from build123d import *

# Parameters (mm, degrees)
CROQUIS1_R              = 2.75
CROQUIS1_R_2            = 1.75
CROQUIS1_R_3            = 1.747778747
CROQUIS1_R_4            = 7.725412866
SALIENTE_EXTRUIR1_DEPTH = 5
CROQUIS2_R              = 3.175
CROQUIS2_R_2            = 27.5
CORTAR_EXTRUIR1_DEPTH   = 5


with BuildPart() as part:
    # Croquis1 → Saliente-Extruir1 (new body)
    with BuildSketch(Plane.XY):
        Polygon((-28.2, -55.083487529), (-28.2, -31.8), (-4.898409704, -31.8), (-4.898409704, 78.2), (5.101590296, 78.2), (5.101590296, -31.8), (28.2, -31.8), (28.2, -54.916512471), (148.2, -54.916512471), (148.2, -64.916512471), (28.2, -64.916512471), (28.2, -88.2), (-28.2, -88.2), (-28.2, -65.083487529), (-148.2, -65.083487529), (-148.2, -55.083487529), align=None)
        with Locations((-23.57, -36.43)):
            Circle(CROQUIS1_R, mode=Mode.SUBTRACT)
        with Locations((23.57, -36.43)):
            Circle(CROQUIS1_R, mode=Mode.SUBTRACT)
        with Locations((23.57, -83.57)):
            Circle(CROQUIS1_R, mode=Mode.SUBTRACT)
        with Locations((-23.57, -83.57)):
            Circle(CROQUIS1_R, mode=Mode.SUBTRACT)
        with Locations((-15.7, -35.3)):
            Circle(CROQUIS1_R_2, mode=Mode.SUBTRACT)
        with Locations((24.7, -44.3)):
            Circle(CROQUIS1_R_3, mode=Mode.SUBTRACT)
        with Locations((15.7, -84.7)):
            Circle(CROQUIS1_R_2, mode=Mode.SUBTRACT)
        with Locations((-24.7, -75.7)):
            Circle(CROQUIS1_R_2, mode=Mode.SUBTRACT)
        with Locations((0, -60)):
            Circle(CROQUIS1_R_4, mode=Mode.SUBTRACT)
    extrude(amount=SALIENTE_EXTRUIR1_DEPTH)

    # Croquis2 → Cortar-Extruir1 (cut)
    with BuildSketch(Plane.XY.offset(5)):
        with Locations((0.101590296, 70)):
            Circle(CROQUIS2_R)
        with Locations((138.2, -59.916512471)):
            Circle(CROQUIS2_R)
        with Locations((-138.2, -60.083487529)):
            Circle(CROQUIS2_R)
        with Locations((0, -60)):
            Circle(CROQUIS2_R_2)
    extrude(amount=-CORTAR_EXTRUIR1_DEPTH, mode=Mode.SUBTRACT)


solid = part.part
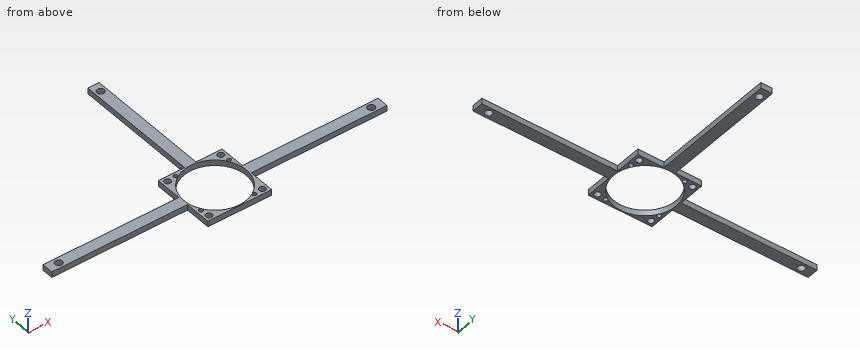
Read the model definition and answer for the solid it produces. Units are mm, in the model's axes. Give positions to 0.01 mm unless a question says otherwise; leave off trailing zeros. Write each loop counter-clockwise with the first axis right and the second up, starting at its lowest first coordinate (ties: lowest second). Pieces come first, ordered by that corner, then holes. Notation, with made-up numbers: (35, 7.5) - (81, 7.5) arc R31 cw to (81, 37.5) - close; hole circle Ø5 at (72, 21.25). An arc over 180 degrees is marked (long way). Use CSV: the item, a comma, the result in double quotes. Start each with the question number.
Item 1: The part is cut by section B-B, the plane z = 2.9. Count the separate pieces of the cut face and the enclosed holes in it, and give its area (3 significant figures).
Item 2: Flat-ended cylindrical pins translate along their axes: P1, Ø1, axis at y = 30.5, z = 1, coming from the -X side; P2, Ø1.5, axis at y = -39, z = 2, coming from the -X side; P3, Ø1.5, axis at x = -72, z = 2, coming from the +Y side. Find the tip coordinate at first contact, or state that the pin passes through.
Item 3: The part is cut by section A-A, the plane y = 70. Give the vertices of the cut face in (x, z).
Item 4: The part is cut by section C-C, the plane x = 0. Give the vertices of the cut face in (y, z), and give its area (3 significant figures).
Item 5: The part is cut by section D-D, the plane x = 96.5. Give the vertices of the cut face in (y, z).
Item 6: Consider line 1 (Y direction, x = 0, z = 1.4); line 2 (Y direction, x = -23.57, z = 2.1); line 3 (Y direction, x = -18, z = 1.1). Determine where each line is inside the solid, lowest interval first.
Taken from the geometry:
1,separate pieces,"1"
1,enclosed holes,"12"
1,area,"4,080 mm2"
2,P1,"x = -4.9"
2,P2,"x = -28.2"
2,P3,"y = -55.08"
3,outline,"(-4.9, 0) - (-3.07, 0) - (-3.07, 5) - (-4.9, 5) - close; (3.28, 0) - (5.1, 0) - (5.1, 5) - (3.28, 5) - close"
4,outline,"(-88.2, 0) - (-87.5, 0) - (-87.5, 5) - (-88.2, 5) - close; (-32.5, 0) - (66.83, 0) - (66.83, 5) - (-32.5, 5) - close; (73.17, 0) - (78.2, 0) - (78.2, 5) - (73.17, 5) - close"
4,area,"525 mm2"
5,outline,"(-64.92, 0) - (-54.92, 0) - (-54.92, 5) - (-64.92, 5) - close"
6,line 1,"-88.2 to -87.5, -32.5 to 66.83, 73.17 to 78.2"
6,line 2,"-88.2 to -86.32, -80.82 to -77.04, -74.36 to -74.17, -45.83 to -39.18, -33.68 to -31.8"
6,line 3,"-88.2 to -80.79, -39.21 to -31.8"
